Geometry check sheet. Reference: the model listing, model coordinates, mm. A direction names the side the tool comes from. Round coordinates to 2 decimals unless told otherwise and drop trailing zeros. Order: outer loops, then holes, each group sorted by start corner. A loop starts at its lowest first (then second) coordinate and runs counter-clockwise, first axis right, second up. Notation, with made-up numbers: (12, 6) - (35, 6) arc R28 cw to (35, 29) - close; hole circle Ø2 at (-5.5, 6.5). An arc over 180 degrees is marked (long way). Use a Markdown table: item, result. Add a question column.
(1) Section check C-C on z = 86. Record the boundary of the cut face in (x, y), then the cut area to 3 significant figures.
(2) Access from +Z, -Z, +X, -X, +Y, -Y to the whole of each face (thin tool, end or side, straight path). Record for faces 1 (the face through (4, 83, 49)), 2 (the face through (51, 83, 4)), 3 (the face through (75, 77, 50)), 4 (the face through (96.5, 83.7, 49.4)).
(3) Gauge pin test, flat ends, axial feed: P1, Ø2.5, axis at y = 38, z = 22.5, coming from the +X side; P2, Ø2.5, axis at x = 78, y = 62.5, coming from the +Z side; P3, Ø1.5, axis at x = 77.5, y = 77.5, coming from the +Z side. Record the tip position at first contact, or that the pin passes through.
(4) Section check D-D on y = 89.5. Record the boundary of the cut face in (x, z), then the cut area to 3 significant figures.
(5) Thickness scan on line 1 along Y through (x, z) = (86, 35.5); line 2 along Y through (x, z) = (40, 85); line 3 along X through (y, z) = (27, 8). Record the ranges inside material, lowest first. Write a range as [from, to].
(6) Mould release check, pull along Z, two halves, no side actions. Record for faces 5 (the face through (83, 49, 4)), 6 (the face through (23, 25, 50)), 7 (the face through (4, 51, 83)), 8 (the face through (50, 75, 23)): released by +Z, released by -Z, zero draft, split by the parting line, or undercut.
(7) Section check A-A on x = 62.5. Record the boundary of the cut face in (y, z), then the cut area to 3 significant figures.
Autodesk Fusion 360 part; units mm, degrees
sketch "Sketch1" plane through (0, 0, 0) normal (0, 0, 1) x (1, 0, 0)
  line L0 (0, 0) -> (100, 0)
  line L1 (100, 0) -> (100, 100)
  line L2 (100, 100) -> (0, 100)
  line L3 (0, 100) -> (0, 0)
extrude "Extrude1" add sketch "Sketch1" along normal blind 100
sketch "Sketch2" plane through (0, 0, 100) normal (0, 0, 1) x (-1, 0, 0)
  line L0 (0, -100) -> (0, 0)
  line L1 (0, 0) -> (-100, 0)
  line L2 (-100, 0) -> (-100, -100)
  line L3 (-100, -100) -> (0, -100)
  line L4 (-25, -75) -> (-75, -75)
  line L5 (-75, -75) -> (-75, -25)
  line L6 (-75, -25) -> (-25, -25)
  line L7 (-25, -25) -> (-25, -75)
extrude "Extrude2" cut sketch "Sketch2" against normal blind 100 contours L4 L5 L6 L7
sketch "Sketch3" plane through (0, 0, 0) normal (0, -1, 0) x (1, 0, 0)
  line L0 (0, 0) -> (100, 0)
  line L1 (100, 0) -> (100, 100)
  line L2 (100, 100) -> (0, 100)
  line L3 (0, 100) -> (0, 0)
  line L4 (25, 75) -> (75, 75)
  line L5 (75, 75) -> (75, 25)
  line L6 (75, 25) -> (25, 25)
  line L7 (25, 25) -> (25, 75)
extrude "Extrude3" cut sketch "Sketch3" against normal blind 100 contours L4 L5 L6 L7
sketch "Sketch4" plane through (100, 0, 0) normal (1, 0, 0) x (0, 1, 0)
  line L0 (0, 0) -> (100, 0)
  line L1 (100, 0) -> (100, 100)
  line L2 (100, 100) -> (0, 100)
  line L3 (0, 100) -> (0, 0)
  line L4 (25, 75) -> (75, 75)
  line L5 (75, 75) -> (75, 25)
  line L6 (75, 25) -> (25, 25)
  line L7 (25, 25) -> (25, 75)
extrude "Extrude4" cut sketch "Sketch4" against normal blind 100 contours L4 L5 L6 L7
fillet "Fillet1" radius 20 12 edges at (75, 50, 100) (50, 25, 100) (50, 75, 100) (25, 50, 100) (50, 100, 25) (75, 100, 50) (50, 100, 75) (25, 100, 50) (0, 50, 25) (0, 25, 50) (0, 50, 75) (0, 75, 50)
fillet "Fillet2" radius 20 12 edges at (50, 0, 75) (25, 0, 50) (50, 0, 25) (75, 0, 50) (100, 50, 75) (100, 25, 50) (100, 75, 50) (100, 50, 25) (75, 50, 0) (50, 25, 0) (25, 50, 0) (50, 75, 0)
Check sheet entries:
| question | item | result |
|---|---|---|
| 1 | outline | (0, 0) - (5, 0) arc R20 ccw to (14, 2.14) - (86, 2.14) arc R20 ccw to (95, 0) - (100, 0) - (100, 5) arc R20 ccw to (97.86, 14) - (97.86, 86) arc R20 ccw to (100, 95) - (100, 100) - (95, 100) arc R20 ccw to (86, 97.86) - (14, 97.86) arc R20 ccw to (5, 100) - (0, 100) - (0, 95) arc R20 ccw to (2.14, 86) - (2.14, 14) arc R20 ccw to (0, 5) - close; hole (24.08, 24.08) - (75.92, 24.08) - (75.92, 75.92) - (24.08, 75.92) - close |
| 1 | area | 6,650 mm2 |
| 2 | face 1 | -X |
| 2 | face 2 | -Z |
| 2 | face 3 | +Y, -Y |
| 2 | face 4 | +X |
| 3 | P1 | stops at x = 91.66 |
| 3 | P2 | stops at z = 92.33 |
| 3 | P3 | stops at z = 90.93 |
| 4 | outline | (0, 0) - (5, 0) arc R20 ccw to (10.5, 0.77) - (89.5, 0.77) arc R20 ccw to (95, 0) - (100, 0) - (100, 5) arc R20 ccw to (99.23, 10.5) - (99.23, 89.5) arc R20 ccw to (100, 95) - (100, 100) - (95, 100) arc R20 ccw to (89.5, 99.23) - (10.5, 99.23) arc R20 ccw to (5, 100) - (0, 100) - (0, 95) arc R20 ccw to (0.77, 89.5) - (0.77, 10.5) arc R20 ccw to (0, 5) - close; hole (22.6, 22.6) - (77.4, 22.6) - (77.4, 77.4) - (22.6, 77.4) - close |
| 4 | area | 6,740 mm2 |
| 5 | line 1 | y = [2.14, 24.08], [75.92, 97.86] |
| 5 | line 2 | y = [2.68, 24.36], [75.64, 97.32] |
| 5 | line 3 | x = [0.23, 21], [79, 99.77] |
| 6 | face 5 | released by -Z |
| 6 | face 6 | undercut |
| 6 | face 7 | undercut |
| 6 | face 8 | zero draft |
| 7 | outline | (0, 0) - (5, 0) arc R20 ccw to (25, 20) - (25, 25) - (20, 25) arc R20 ccw to (0, 5) - close; (0, 95) arc R20 ccw to (20, 75) - (25, 75) - (25, 80) arc R20 ccw to (5, 100) - (0, 100) - close; (75, 20) arc R20 ccw to (95, 0) - (100, 0) - (100, 5) arc R20 ccw to (80, 25) - (75, 25) - close; (75, 75) - (80, 75) arc R20 ccw to (100, 95) - (100, 100) - (95, 100) arc R20 ccw to (75, 80) - close |
| 7 | area | 1,810 mm2 |
